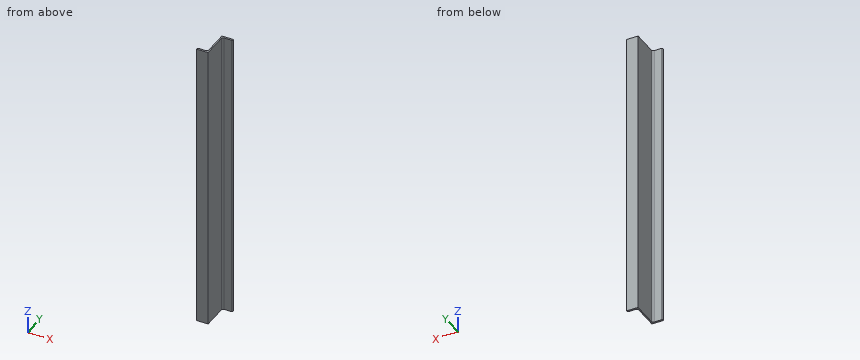
Autodesk Inventor part; units mm, degrees
ref_plane "Start plane" through (0, 0, 80) normal (0, 0, 1) x (1, 0, 0)
ref_plane "End plane" through (0, 0, 2120) normal (0, 0, 1) x (1, 0, 0)
ref_plane "Work Plane4" through (-1500, 0, 80) normal (0, 0, -1) x (-1, 0, 0)
ref_plane "Start plane" through (0, 0, 80) normal (0, 0, 1) x (1, 0, 0)
ref_plane "End plane" through (0, 0, 2120) normal (0, 0, 1) x (1, 0, 0)
sketch "Sketch" plane through (0, 0, 0) normal (0, 0, 1) x (1, 0, 0)
  line L0 (-75, -100) -> (5, -100)
  line L1 (5, -100) -> (5, 74)
  line L2 (18, 87) -> (68.5, 87)
  line L3 (75, 93.5) -> (75, 100)
  line L4 (75, 100) -> (-5, 100)
  line L5 (-5, 100) -> (-5, -74)
  line L6 (-18, -87) -> (-68.5, -87)
  line L7 (-75, -93.5) -> (-75, -100)
  line L8 (173.6154, 0) -> (-40.1539, 0) construction
  line L9 (0, -212) -> (0, 68) construction
  arc A0 (-18, -87) -> (-5, -74) centre (-18, -74) ccw
  arc A1 (18, 87) -> (5, 74) centre (18, 74) ccw
  arc A2 (-68.5, -87) -> (-75, -93.5) centre (-68.5, -93.5) ccw
  arc A3 (68.5, 87) -> (75, 93.5) centre (68.5, 93.5) ccw
  line L10 (0, 162.4) -> (0, -274.4) construction
  line L11 (-126.3385, 0) -> (223.6078, 0) construction
  point P0 (5, 87)
  point P1 (75, 87)
  point P2 (-5, -87)
  point P3 (-75, -87)
  dimension "d0" = 200
  dimension "d1" = 80
  dimension "d2" = 80
  dimension "d3" = 13
  dimension "d4" = 13
  dimension "d5" = 10
  dimension "d10" = 13
  dimension "d11" = 6.5
  dimension "d12" = 5
  dimension "d13" = 100
extrude "Body" add sketch "Sketch" along normal up to surface (2040 mm away) from surface at 80
sketch "Sketch3" plane through (0, 0, 0) normal (0, 0, 1) x (1, 0, 0)
  line L0 (0, 0) -> (10, 0)
ref_plane "Work Plane3" through (0, 0, 0) normal (0, -1, 0) x (1, 0, 0)
sketch "Sketch4" plane through (0, 0, 0) normal (0, -1, 0) x (1, 0, 0)
  line L0 (-2, 80) -> (12, 80)
  line L1 (-2, 2120) -> (12, 2120)
  dimension "d17" = 2040
ref_plane "Work Plane4" through (-1500, 0, 80) normal (0, 0, -1) x (-1, 0, 0)
split "Split1" plane through (-1500, 0, 80) removes the side toward (0, 0, -1)
ref_plane "Work Plane5" through (3500, 0, 2120) normal (0, 0, 1) x (1, 0, 0)
split "Split2" plane through (3500, 0, 2120) removes the side toward (0, 0, 1)
equation "\"d0\" = G_H"
equation "\"d1\" = G_W"
equation "\"d2\" = G_W"
equation "\"d3\" = G_T1"
equation "\"d4\" = G_T1"
equation "\"d5\" = G_T"
equation "\"d10\" = G_IR"
equation "\"d11\" = G_ER"
equation "\"d12\" = 0.5 * d5"
equation "\"d13\" = 0.5 * d0"
equation "\"d6\" = G_L"
equation "\"G_W\" = 80"
equation "\"G_H\" = 200"
equation "\"G_T\" = 10"
equation "\"G_T1\" = 13"
equation "\"G_IR\" = 13"
equation "\"G_ER\" = 6.5"
equation "\"G_L\" = d17"
properties part number "DIN1027 - Z 200 - 2040" material "Steel, Mild"
Can you work these out from the model? Positions are in its coordinate system, mm. Give positions to 0.01 mm unless a question says otherwise; leave off trailing zeros. Loops run counter-clockwise (first coordinate to the right, second up) from the corner with the lowest first, then second, coordinate; pieces in that order, holes last. Notation, with made-up numbers: M 65,-13.5 L 117,-13.5 A10 cw 117,-9.5 Z; hole C -8,-21.5 d1. An arc over 180 degrees is marked long. One line per item, written item: value.
(1) Suppose I cut it at A-A on z = 1114. List the corners of the cut face in (x, y) for me, plus the area to 3 significant figures.
Returned:
outline: M -75,-100 L 5,-100 L 5,74 A13 cw 18,87 L 68.5,87 A6.5 ccw 75,93.5 L 75,100 L -5,100 L -5,-74 A13 cw -18,-87 L -68.5,-87 A6.5 ccw -75,-93.5 Z
area: 3,870 mm^2
(2) Will these pins go through, and if not, where does the flat tip stop? pin 1 (6 mm diameter, centred on y = 56, z = 1517, fed in from -X); pin 2 (3 mm diameter, centred on y = -41, z = 989, fed in from +X); pin 3 (10 mm diameter, centred on x = -48.5, z = 1360.5, fed in from +Y).
Returned:
pin 1: x = -5
pin 2: x = 5
pin 3: y = -87
(3) I need wall thicknesses on line 1 (X direction, y = 17, z = 1405); line 2 (Y direction, x = 25.5, z = 1617); line 3 (Y direction, x = -18.5, z = 1408.5). Which ranges of each line are inside material? Lowest first, please.
Returned:
line 1: -5 to 5
line 2: 87 to 100
line 3: -100 to -87
(4) Suppose I cut it at C-C on x = 51. List the corners of the cut face in (y, z) for me.
Returned:
outline: M 87,80 L 100,80 L 100,2120 L 87,2120 Z
(5) Suppose I cut it at B-B on y = -33. List the corners of the cut face in (x, z) for me.
Returned:
outline: M -5,80 L 5,80 L 5,2120 L -5,2120 Z
